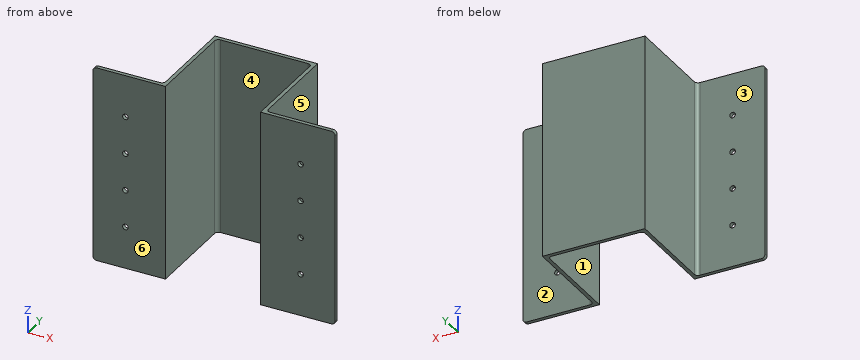
```python
from build123d import *

# Parameters (mm, degrees)
BOSS_EXTRUDE1_DEPTH = 105
FILLET2_R           = 2
FILLET3_R           = 2
FILLET4_R           = 2
FILLET5_R           = 2
SKETCH2_R           = 1.5
CUT_EXTRUDE1_DEPTH  = 105
FILLET6_R           = 2


with BuildPart() as part:
    # Sketch1 → Boss-Extrude1 (new body)
    with BuildSketch(Plane.XY):
        Polygon((-42.084779145, 1.426065285), (8.915220855, 1.426065285), (8.915220855, -49.573934715), (48.915220855, -49.573934715), (48.915220855, -47.573934715), (10.915220855, -47.573934715), (10.915220855, 3.426065285), (-44.084779145, 3.426065285), (-44.084779145, -47.573934715), (-80.999498671, -47.573934715), (-80.999498671, -49.573934715), (-42.084779145, -49.573934715), align=None)
    extrude(amount=BOSS_EXTRUDE1_DEPTH)

    # Fillet2
    fillet2_edges = [part.edges().sort_by_distance(p)[0] for p in [
        (-44.084779145, -47.573934715, 52.5),
    ]]
    fillet(fillet2_edges, radius=FILLET2_R)

    # Fillet3
    fillet3_edges = [part.edges().sort_by_distance(p)[0] for p in [
        (-42.084779145, 1.426065285, 52.5),
    ]]
    fillet(fillet3_edges, radius=FILLET3_R)

    # Fillet4
    fillet4_edges = [part.edges().sort_by_distance(p)[0] for p in [
        (8.915220855, 1.426065285, 52.5),
    ]]
    fillet(fillet4_edges, radius=FILLET4_R)

    # Fillet5
    fillet5_edges = [part.edges().sort_by_distance(p)[0] for p in [
        (10.915220855, -47.573934715, 52.5),
    ]]
    fillet(fillet5_edges, radius=FILLET5_R)

    # Sketch2 → Cut-Extrude1 (cut)
    with BuildSketch(Plane(origin=(0, -47.573934715, 0), x_dir=(1, 0, 0), z_dir=(0, 1, 0))):
        with Locations((-63.542138908, -42.5)):
            Circle(SKETCH2_R)
        with Locations((-63.542138908, -22.5)):
            Circle(SKETCH2_R)
        with Locations((-63.542138908, -82.5)):
            Circle(SKETCH2_R)
        with Locations((-63.542138908, -62.5)):
            Circle(SKETCH2_R)
        with Locations((30.372580618, -82.5)):
            Circle(SKETCH2_R)
        with Locations((30.372580618, -62.5)):
            Circle(SKETCH2_R)
        with Locations((30.372580618, -42.5)):
            Circle(SKETCH2_R)
        with Locations((30.372580618, -22.5)):
            Circle(SKETCH2_R)
    extrude(amount=-CUT_EXTRUDE1_DEPTH, mode=Mode.SUBTRACT)

    # Fillet6
    fillet6_edges = [part.edges().sort_by_distance(p)[0] for p in [
        (-80.999498671, -48.573934715, 0),
        (48.915220855, -48.573934715, 0),
        (48.915220855, -48.573934715, 105),
        (-80.999498671, -48.573934715, 105),
    ]]
    fillet(fillet6_edges, radius=FILLET6_R)


solid = part.part
```
Geometry: final body of the model. Coordinates: model frame, mm. Face numbers are marked on the shaded views. A direction names the side the tool comes from. Coordinates: 2 decimals unless noted, no trailing zeros. Loops run counter-clockwise (first coordinate to the right, second up) from the corner with the lowest first, then second, coordinate; pieces in that order, holes last. Notation, with made-up numbers: (53, 68) -> (98, 68) arc R30 ccw to (98, 101) -> close; hole circle Ø3 at (72.25, 17). An arc over 180 degrees is marked (long way). Use a Markdown table: item, result. Add a question column.
(1) Pin query (flat end, axial travel): pin 1 Ø2.5 at (x, z) = (30.37, 42.5) entering from +Y; pin 2 Ø24.5 at (y, z) = (-29, 32) entering from +X; pin 3 Ø12 at (y, z) = (-7.5, 50) entering from -X; pin 4 Ø3.5 at (x, z) = (30.37, 22.5) entering from +Y. Return the tip coordinate at first contact, or that it passes through.
(2) Section query A-A, the plane y = -20. Return loops of the section in (x, z).
(3) Section query D-D, the plane x = 1.5. Return loops of the section in (y, z), plus the area to 3 significant figures.
(4) Section query C-C, the plane z = 87. Return loops of the section in (x, y).
(5) Access query for the marked faces 1, 2 and 3. Directions: +Z, -Z, +X, -X, +Y, -Y. A direction counts if a zero-diameter tool reaches every point of the face in a straight line with its end or side. Return the directions, or none.
(6) Mould query, pull axis X, two halves, no side actions, for the marked faces 4, 5 and 6. Classes: pulls with the +X half, pulls with the -X half, needs draft (parallel to the pull), parting line crosses it, or undercut.
(7) Line query: line 1 along X through (y, z) = (-49, 42.5); line 2 along X through (y, z) = (-4.5, 65); line 3 along Y through (x, z) = (-73, 68). Output: solid intervals per line, ascending.
(8) Section query B-B, the plane z = 42.5. Return loops of the section in (x, y).
Answer:
| question | item | result |
|---|---|---|
| 1 | pin 1 | passes through |
| 1 | pin 2 | stops at x = 10.92 |
| 1 | pin 3 | stops at x = -44.08 |
| 1 | pin 4 | stops at y = -47.57 |
| 2 | outline | (-44.08, 0) -> (-42.08, 0) -> (-42.08, 105) -> (-44.08, 105) -> close; (8.92, 0) -> (10.92, 0) -> (10.92, 105) -> (8.92, 105) -> close |
| 3 | outline | (1.43, 0) -> (3.43, 0) -> (3.43, 105) -> (1.43, 105) -> close |
| 3 | area | 210 mm^2 |
| 4 | outline | (-81, -49.57) -> (-42.08, -49.57) -> (-42.08, -0.57) arc R2 cw to (-40.08, 1.43) -> (6.92, 1.43) arc R2 cw to (8.92, -0.57) -> (8.92, -49.57) -> (48.92, -49.57) -> (48.92, -47.57) -> (12.92, -47.57) arc R2 cw to (10.92, -45.57) -> (10.92, 3.43) -> (-44.08, 3.43) -> (-44.08, -45.57) arc R2 cw to (-46.08, -47.57) -> (-81, -47.57) -> close |
| 5 | face 1 | +Z, -Z, -Y |
| 5 | face 2 | +Z, -Z, +X, +Y |
| 5 | face 3 | +Z, -Z, -X, +Y |
| 6 | face 4 | undercut |
| 6 | face 5 | pulls with the +X half |
| 6 | face 6 | needs draft |
| 7 | line 1 | x = -81 to -65.04, -62.04 to -42.08, 8.92 to 28.87, 31.87 to 48.92 |
| 7 | line 2 | x = -44.08 to -42.08, 8.92 to 10.92 |
| 7 | line 3 | y = -49.57 to -47.57 |
| 8 | outline | (-81, -49.57) -> (-65.04, -49.57) -> (-65.04, -47.57) -> (-81, -47.57) -> close; (-62.04, -49.57) -> (-42.08, -49.57) -> (-42.08, -0.57) arc R2 cw to (-40.08, 1.43) -> (6.92, 1.43) arc R2 cw to (8.92, -0.57) -> (8.92, -49.57) -> (28.87, -49.57) -> (28.87, -47.57) -> (12.92, -47.57) arc R2 cw to (10.92, -45.57) -> (10.92, 3.43) -> (-44.08, 3.43) -> (-44.08, -45.57) arc R2 cw to (-46.08, -47.57) -> (-62.04, -47.57) -> close; (31.87, -49.57) -> (48.92, -49.57) -> (48.92, -47.57) -> (31.87, -47.57) -> close |
